Can you work these out from the model? Positions are in its coordinate system, mm. Face numbers are marked on the shaded views. A direction names the side the tool comes from. Give positions to 0.01 mm unless a question says otherwise; leave off trailing zeros. Loops run counter-clockwise (first coordinate to the right, second up) from the corner with the lowest first, then second, coordinate; pieces in that order, holes last. Notation, with made-up numbers: (29, 41.5) - (79, 41.5) arc R16 ccw to (79, 55.5) - close; hole circle Ø5 at (23, -38). An arc over 180 degrees is marked (long way). Use a Markdown table: item, result. Add a question column.
```python
from build123d import *

# Parameters (mm, degrees)
BOSS_EXTRUDE1_DEPTH      = 70
BOSS_EXTRUDE1_2_DEPTH    = 70
SKETCH3_R                = 5
BOSS_EXTRUDE3_DEPTH      = 12
SKETCH4_R                = 5
BOSS_EXTRUDE4_DEPTH      = 12
BOSS_EXTRUDE5_REACH      = 98.366
SKETCH5_W                = 12
SKETCH5_H                = 30
BOSS_EXTRUDE6_REACH      = 98.366
SKETCH6_W                = 12
SKETCH6_H                = 30
BOSS_EXTRUDE7_DEPTH      = 35
BOSS_EXTRUDE7_DEPTH_BACK = 35
SKETCH8_R                = 7.5
CUT_EXTRUDE1_DEPTH       = 132.745671501
CUT_EXTRUDE4_DEPTH       = 122.337535907
CUT_EXTRUDE5_DEPTH       = 122.337535907
SKETCH12_R               = 15
CUT_EXTRUDE6_DEPTH       = 5
SKETCH13_R               = 5
CUT_EXTRUDE7_DEPTH       = 118.019851709


with BuildPart() as part:
    # Sketch2 → Boss-Extrude1 (new body)
    with BuildSketch(Plane(origin=(0, 0, 0), x_dir=(1, 0, 0), z_dir=(0, 1, 0))):
        with BuildLine():
            Line((-29.849623113, 3), (-22.299103121, 3))
            ThreePointArc((-22.299103121, 3), (-1.510093754, 22.449267624), (21.696428571, 5.959445213))
            ThreePointArc((21.696428571, 5.959445213), (25.319689527, 7.44207783), (29.196428571, 6.896996352))
            ThreePointArc((29.196428571, 6.896996352), (-1.975679862, 29.934874128), (-29.849623113, 3))
        make_face()
    extrude(amount=BOSS_EXTRUDE1_DEPTH)

    # Sketch6 → Boss-Extrude6 (add, up to next)
    with BuildSketch(Plane(origin=(-29.849623113, 0, 0), x_dir=(0, 0, -1), z_dir=(1, 0, 0)), mode=Mode.PRIVATE) as boss_extrude6_sk1:
        with Locations((9, 55)):
            Rectangle(SKETCH6_W, SKETCH6_H)
    boss_extrude6_tool1 = extrude(boss_extrude6_sk1.sketch, amount=BOSS_EXTRUDE6_REACH, mode=Mode.PRIVATE) - part.part


with BuildPart() as body_2:
    # Sketch2 → Boss-Extrude1 2 (new body)
    with BuildSketch(Plane(origin=(0, 0, 0), x_dir=(1, 0, 0), z_dir=(0, 1, 0))):
        with BuildLine():
            Line((-29.849623113, -3), (-22.299103121, -3))
            ThreePointArc((-22.299103121, -3), (-1.510093754, -22.449267624), (21.696428571, -5.959445213))
            ThreePointArc((21.696428571, -5.959445213), (25.319689527, -7.44207783), (29.196428571, -6.896996352))
            ThreePointArc((29.196428571, -6.896996352), (-1.975679862, -29.934874128), (-29.849623113, -3))
        make_face()
    extrude(amount=BOSS_EXTRUDE1_2_DEPTH)

    # Sketch5 → Boss-Extrude5 (add, up to next)
    with BuildSketch(Plane(origin=(-29.849623113, 0, 0), x_dir=(0, 0, -1), z_dir=(1, 0, 0)), mode=Mode.PRIVATE) as boss_extrude5_sk1:
        with Locations((-9, 55)):
            Rectangle(SKETCH5_W, SKETCH5_H)
    boss_extrude5_tool1 = extrude(boss_extrude5_sk1.sketch, amount=BOSS_EXTRUDE5_REACH, mode=Mode.PRIVATE) - body_2.part


with BuildPart() as body_3:
    # Sketch3 → Boss-Extrude3 (new body)
    with BuildSketch(Plane.XY.offset(-3)):
        with BuildLine():
            Line((-29.849623113, 70), (-44.849623113, 70))
            ThreePointArc((-44.849623113, 70), (-59.849623113, 55), (-44.849623113, 40))
            Line((-44.849623113, 40), (-29.849623113, 40))
            Line((-29.849623113, 40), (-29.849623113, 70))
        make_face()
        with Locations((-44.849623113, 55)):
            Circle(SKETCH3_R, mode=Mode.SUBTRACT)
    extrude(amount=-BOSS_EXTRUDE3_DEPTH)


with BuildPart() as body_4:
    # Sketch4 → Boss-Extrude4 (new body)
    with BuildSketch(Plane(origin=(0, 0, 3), x_dir=(-1, 0, 0), z_dir=(0, 0, -1))):
        with BuildLine():
            Line((29.849623113, 40), (29.849623113, 70))
            Line((29.849623113, 70), (44.849623113, 70))
            ThreePointArc((44.849623113, 70), (59.849623113, 55), (44.849623113, 40))
            Line((44.849623113, 40), (29.849623113, 40))
        make_face()
        with Locations(Location((44.849623113, 55, 0), (0, 0, 180))):
            Circle(SKETCH4_R, mode=Mode.SUBTRACT)
    extrude(amount=-BOSS_EXTRUDE4_DEPTH)


with BuildPart() as body_2_1:
    add(body_2.part)

    add(body_4.part)  # Boss-Extrude5 merges body 4
    add(boss_extrude5_tool1.solids().sort_by_distance((-29.849623, 55, 9))[0])


with BuildPart() as part_1:
    add(part.part)

    add(body_3.part)  # Boss-Extrude6 merges body 3
    add(boss_extrude6_tool1.solids().sort_by_distance((-29.849623, 55, -9))[0])


    add(body_2_1.part)  # Boss-Extrude7 merges body 2
    # Sketch7 → Boss-Extrude7 (add, two sides: drawn at the far end of the back side and taken through both)
    with BuildSketch(Plane.XY.offset(-BOSS_EXTRUDE7_DEPTH_BACK)):
        with BuildLine():
            Line((99.980762114, 9.607695155), (70.811589784, 26.448524651))
            ThreePointArc((70.811589784, 26.448524651), (30.514428415, 46.25), (67.811589784, 21.252372228))
            Line((67.811589784, 21.252372228), (96.980762114, 4.411542732))
            Line((96.980762114, 4.411542732), (90.980762114, -5.980762114))
            Line((90.980762114, -5.980762114), (65, 9.019237886))
            ThreePointArc((65, 9.019237886), (24.019237886, 50), (80, 35))
            Line((80, 35), (105.980762114, 20))
            Line((105.980762114, 20), (99.980762114, 9.607695155))
        make_face()
    extrude(amount=BOSS_EXTRUDE7_DEPTH + BOSS_EXTRUDE7_DEPTH_BACK)

    # Sketch8 → Cut-Extrude1 (cut, through all)
    with BuildSketch(Plane(origin=(0, 0, 0), x_dir=(1, 0, 0), z_dir=(0, 1, 0))):
        with Locations((26.25, 0)):
            Circle(SKETCH8_R)
    extrude(amount=CUT_EXTRUDE1_DEPTH, mode=Mode.SUBTRACT)

    # Sketch10 → Cut-Extrude4 (cut, through all)
    with BuildSketch(Plane(origin=(35.155444566, 60.891016151, 0), x_dir=(0.8660254037844384, -0.5000000000000007, 0), z_dir=(0.5000000000000006, 0.8660254037844383, 0))):
        with BuildLine():
            Line((66.782032303, 15), (51.782032303, 15))
            Line((51.782032303, 15), (51.782032303, 35))
            Line((51.782032303, 35), (81.782032303, 35))
            Line((81.782032303, 35), (81.782032303, 0))
            ThreePointArc((81.782032303, 0), (77.388634021, 10.606601718), (66.782032303, 15))
        make_face()
    extrude(amount=-CUT_EXTRUDE4_DEPTH, mode=Mode.SUBTRACT)

    # Sketch11 → Cut-Extrude5 (cut, through all)
    with BuildSketch(Plane(origin=(35.155444566, 60.891016151, 0), x_dir=(0.8660254037844384, -0.5000000000000007, 0), z_dir=(0.5000000000000006, 0.8660254037844383, 0))):
        with BuildLine():
            Line((66.782032303, -15), (51.782032303, -15))
            Line((51.782032303, -15), (51.782032303, -35))
            Line((51.782032303, -35), (81.782032303, -35))
            Line((81.782032303, -35), (81.782032303, 0))
            ThreePointArc((81.782032303, 0), (77.388634021, -10.606601718), (66.782032303, -15))
        make_face()
    extrude(amount=-CUT_EXTRUDE5_DEPTH, mode=Mode.SUBTRACT)

    # Sketch12 → Cut-Extrude6 (cut)
    with BuildSketch(Plane(origin=(35.155444566, 60.891016151, 0), x_dir=(0.8660254037844384, -0.5000000000000007, 0), z_dir=(0.5000000000000006, 0.8660254037844383, 0))):
        with Locations((66.782032303, 0)):
            Circle(SKETCH12_R)
    extrude(amount=-CUT_EXTRUDE6_DEPTH, mode=Mode.SUBTRACT)

    # Sketch13 → Cut-Extrude7 (cut, through all)
    with BuildSketch(Plane(origin=(32.655444566, 56.560889132, 0), x_dir=(0.8660254037844383, -0.5000000000000008, 0), z_dir=(0.5000000000000007, 0.8660254037844382, 0))):
        with Locations(Location((66.782032303, 0, 0), (0, 0, 180))):
            Circle(SKETCH13_R)
    extrude(amount=-CUT_EXTRUDE7_DEPTH, mode=Mode.SUBTRACT)


solid = part_1.part
```
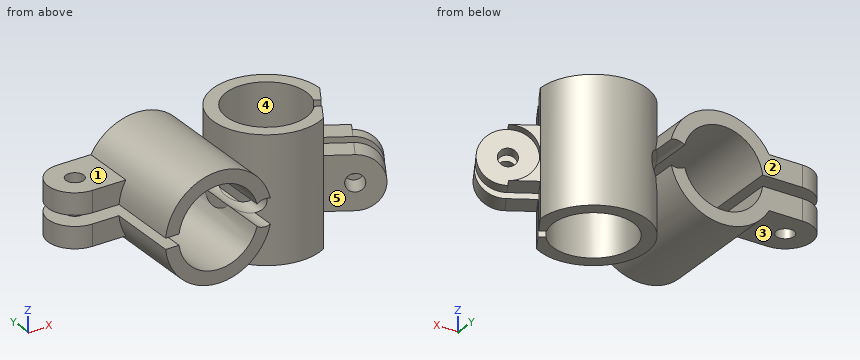
1. Suppose I cut it at B-B (z = -20). List the corners of the cut face in (x, y) for me, and give its area (3 significant figures).
2. On a 3-axis mill with a long thin cutter (end or side, diameter ignored), from which of +Z, -Z, +X, -X, +Y, -Y can I reach the whole of each face in a straight line? I mean the marked faces 1 and 2. Say none if no direction works.
3. Suppose I cut it at A-A (x = 50). List the corners of the cut face in (y, z) for me.
4. Suppose I cut it at C-C (y = 55). List the corners of the cut face in (x, z) for me.
5. Will these pins go through, and if not, where does the flat tip stop? P1, Ø4, axis at x = 38.5, z = -10, coming from the +Y side; P2, Ø9.5, axis at x = -36, z = -11, coming from the -Y side; P3, Ø21.5, axis at x = 7.5, z = 12.5, coming from the -Y side.
6. If we mould it in two halves opening along Y, with no side actions, what happens to the marked faces 3, 4 and 5? For each: released by +Y, released by -Y, zero draft, split by the parting line, or undercut.
7. Please list where these lines run through material, in increasing order: line 1 along Z through (x, y) = (-30, 44); line 2 along X through (y, z) = (52, 20.5); line 3 along X through (y, z) = (34.5, 23). Write a range as [from, to].
8. Suppose I cut it at D-D (x = -15.5). List the corners of the cut face in (y, z) for me, and give its area (3 significant figures).
Results below:
| question | item | result |
|---|---|---|
| 1 | outline | (-22.36, 0) - (-10.31, 0) - (-10.31, 70) - (-22.36, 70) - close; (10.31, 0) - (22.36, 0) - (22.36, 23.34) arc R30 ccw to (65, 9.02) - (71, 19.41) - (67.81, 21.25) arc R22.5 cw (long way) to (70.81, 26.45) - (74, 24.61) - (80, 35) arc R30 ccw to (22.36, 46.66) - (22.36, 70) - (10.31, 70) - close |
| 1 | area | 2,780 mm² |
| 2 | face 1 | +Z, -X, +Y, -Y |
| 2 | face 2 | +Z, -Z, +X, -X, +Y |
| 3 | outline | (5, -35) - (12.5, -35) - (12.5, 35) - (5, 35) - close; (57.5, -35) - (65, -35) - (65, 35) - (57.5, 35) - close |
| 4 | outline | (-59.85, -15) - (-49.85, -15) - (-49.85, -3) - (-59.85, -3) - close; (-59.85, 3) - (-49.85, 3) - (-49.85, 15) - (-59.85, 15) - close; (-39.85, -15) - (-25.98, -15) arc R30 ccw to (27.64, -11.66) - (27.64, -35) - (39.69, -35) - (39.69, 35) - (27.64, 35) - (27.64, 11.66) arc R30 ccw to (-25.98, 15) - (-39.85, 15) - (-39.85, 3) - (-22.3, 3) arc R22.5 cw to (21.7, 5.96) arc R7.5 cw (long way) to (21.7, -5.96) arc R22.5 cw to (-22.3, -3) - (-39.85, -3) - close; (60.31, -35) - (72.36, -35) - (72.36, 35) - (60.31, 35) - close |
| 5 | P1 | y = 63.46 |
| 5 | P2 | y = 40 |
| 5 | P3 | y = 0 |
| 6 | face 3 | zero draft |
| 6 | face 4 | undercut |
| 6 | face 5 | released by -Y |
| 7 | line 1 | [-15, -3], [3, 15] |
| 7 | line 2 | [-21.9, -9.27], [9.27, 21.9], [25.28, 35.26], [64.74, 74.72] |
| 7 | line 3 | [-19.26, 19.26], [20, 27.51], [72.49, 79.71] |
| 8 | outline | (0, -25.69) - (70, -25.69) - (70, -16.31) - (0, -16.31) - close; (0, 16.31) - (70, 16.31) - (70, 25.69) - (0, 25.69) - close |
| 8 | area | 1,310 mm² |
